The listing builds one solid part. Answer for the finished solid, in the listing's coordinates (mm). Coordinates: 2 decimals unless noted, no trailing zeros. Order: outer loops, then holes, each group sorted by start corner. A loop starts at its lowest first (then second) coordinate and runs counter-clockwise, first axis right, second up. Notation, with made-up numbers: (33, 55.5) -> (74, 55.5) arc R28 cw to (74, 81.5) -> close; hole circle Ø10 at (-3.5, 62.5). An arc over 180 degrees is marked (long way). Return JSON: item names as keys, results as strings.
```python
from build123d import *

# Parameters (mm, degrees)
F0_R     = 7.5
F1_DEPTH = 20


with BuildPart() as f1:
    # F0 (on Top) → F1 (new body)
    with BuildSketch(Plane.XY):
        with BuildLine():
            Line((-13.784993, 1.235994), (-16.59268, 2.329543))
            ThreePointArc((-16.59268, 2.329543), (-20, 0), (-16.59268, -2.329543))
            Line((-16.59268, -2.329543), (-13.784993, -1.235994))
            ThreePointArc((-13.784993, -1.235994), (-11.769423, -2.341084), (-13.208667, -4.133379))
            Line((-13.208667, -4.133379), (-16.221115, -4.197527))
            ThreePointArc((-16.221115, -4.197527), (-18.477591, -7.653669), (-14.43816, -8.501961))
            Line((-14.43816, -8.501961), (-12.262679, -6.417198))
            ThreePointArc((-12.262679, -6.417198), (-9.977635, -6.666843), (-10.621442, -8.873483))
            Line((-10.621442, -8.873483), (-13.380032, -10.085561))
            ThreePointArc((-13.380032, -10.085561), (-14.142136, -14.142136), (-10.085561, -13.380032))
            Line((-10.085561, -13.380032), (-8.873483, -10.621442))
            ThreePointArc((-8.873483, -10.621442), (-6.666843, -9.977635), (-6.417198, -12.262679))
            Line((-6.417198, -12.262679), (-8.501961, -14.43816))
            ThreePointArc((-8.501961, -14.43816), (-7.653669, -18.477591), (-4.197527, -16.221115))
            Line((-4.197527, -16.221115), (-4.133379, -13.208667))
            ThreePointArc((-4.133379, -13.208667), (-2.341084, -11.769423), (-1.235994, -13.784993))
            Line((-1.235994, -13.784993), (-2.329543, -16.59268))
            ThreePointArc((-2.329543, -16.59268), (0, -20), (2.329543, -16.59268))
            Line((2.329543, -16.59268), (1.235994, -13.784993))
            ThreePointArc((1.235994, -13.784993), (2.341084, -11.769423), (4.133379, -13.208667))
            Line((4.133379, -13.208667), (4.197527, -16.221115))
            ThreePointArc((4.197527, -16.221115), (7.653669, -18.477591), (8.501961, -14.43816))
            Line((8.501961, -14.43816), (6.417198, -12.262679))
            ThreePointArc((6.417198, -12.262679), (6.666843, -9.977635), (8.873483, -10.621442))
            Line((8.873483, -10.621442), (10.085561, -13.380032))
            ThreePointArc((10.085561, -13.380032), (14.142136, -14.142136), (13.380032, -10.085561))
            Line((13.380032, -10.085561), (10.621442, -8.873483))
            ThreePointArc((10.621442, -8.873483), (9.977635, -6.666843), (12.262679, -6.417198))
            Line((12.262679, -6.417198), (14.43816, -8.501961))
            ThreePointArc((14.43816, -8.501961), (18.477591, -7.653669), (16.221115, -4.197527))
            Line((16.221115, -4.197527), (13.208667, -4.133379))
            ThreePointArc((13.208667, -4.133379), (11.769423, -2.341084), (13.784993, -1.235994))
            Line((13.784993, -1.235994), (16.59268, -2.329543))
            ThreePointArc((16.59268, -2.329543), (20, 0), (16.59268, 2.329543))
            Line((16.59268, 2.329543), (13.784993, 1.235994))
            ThreePointArc((13.784993, 1.235994), (11.769423, 2.341084), (13.208667, 4.133379))
            Line((13.208667, 4.133379), (16.221115, 4.197527))
            ThreePointArc((16.221115, 4.197527), (18.477591, 7.653669), (14.43816, 8.501961))
            Line((14.43816, 8.501961), (12.262679, 6.417198))
            ThreePointArc((12.262679, 6.417198), (9.977635, 6.666843), (10.621442, 8.873483))
            Line((10.621442, 8.873483), (13.380032, 10.085561))
            ThreePointArc((13.380032, 10.085561), (14.142136, 14.142136), (10.085561, 13.380032))
            Line((10.085561, 13.380032), (8.873483, 10.621442))
            ThreePointArc((8.873483, 10.621442), (6.666843, 9.977635), (6.417198, 12.262679))
            Line((6.417198, 12.262679), (8.501961, 14.43816))
            ThreePointArc((8.501961, 14.43816), (7.653669, 18.477591), (4.197527, 16.221115))
            Line((4.197527, 16.221115), (4.133379, 13.208667))
            ThreePointArc((4.133379, 13.208667), (2.341084, 11.769423), (1.235994, 13.784993))
            Line((1.235994, 13.784993), (2.329543, 16.59268))
            ThreePointArc((2.329543, 16.59268), (0, 20), (-2.329543, 16.59268))
            Line((-2.329543, 16.59268), (-1.235994, 13.784993))
            ThreePointArc((-1.235994, 13.784993), (-2.341084, 11.769423), (-4.133379, 13.208667))
            Line((-4.133379, 13.208667), (-4.197527, 16.221115))
            ThreePointArc((-4.197527, 16.221115), (-7.653669, 18.477591), (-8.501961, 14.43816))
            Line((-8.501961, 14.43816), (-6.417198, 12.262679))
            ThreePointArc((-6.417198, 12.262679), (-6.666843, 9.977635), (-8.873483, 10.621442))
            Line((-8.873483, 10.621442), (-10.085561, 13.380032))
            ThreePointArc((-10.085561, 13.380032), (-14.142136, 14.142136), (-13.380032, 10.085561))
            Line((-13.380032, 10.085561), (-10.621442, 8.873483))
            ThreePointArc((-10.621442, 8.873483), (-9.977635, 6.666843), (-12.262679, 6.417198))
            Line((-12.262679, 6.417198), (-14.43816, 8.501961))
            ThreePointArc((-14.43816, 8.501961), (-18.477591, 7.653669), (-16.221115, 4.197527))
            Line((-16.221115, 4.197527), (-13.208667, 4.133379))
            ThreePointArc((-13.208667, 4.133379), (-11.769423, 2.341084), (-13.784993, 1.235994))
        make_face()
        Circle(F0_R, mode=Mode.SUBTRACT)
    extrude(amount=F1_DEPTH)


solid = f1.part
```
Item 1: The part is cut by section D-D on x = 8. Determine the outline of the cut face in (y, z), plus the area to 3 significant figures.
Answer list:
{"outline": "(-18.3, 0) -> (-13.91, 0) -> (-13.91, 20) -> (-18.3, 20) -> close; (-9.81, 0) -> (9.81, 0) -> (9.81, 20) -> (-9.81, 20) -> close; (13.91, 0) -> (18.3, 0) -> (18.3, 20) -> (13.91, 20) -> close", "area": "568 mm2"}
Item 2: Flat-ended cylindrical pins translate along their axes: pin 1 (10 mm diameter, centred on x = -3.5, y = 15.5, fed in from -Z); pin 2 (2 mm diameter, centred on x = -6.5, z = 15.5, fed in from -Y); pin 3 (10 mm diameter, centred on x = -6.5, z = 2.5, fed in from +Y); pin 4 (5 mm diameter, centred on y = 6, z = 15, fed in from -X). Find the tip coordinate at first contact, or state that the pin passes through.
Answer list:
{"pin 1": "z = 0", "pin 2": "y = -18.67", "pin 3": "y = 19.5", "pin 4": "x = -18.67"}
Item 3: The part is cut by section A-A on y = 0. Determine the outline of the cut face in (x, z), plus the area to 3 significant figures.
Answer list:
{"outline": "(-20, 0) -> (-7.5, 0) -> (-7.5, 20) -> (-20, 20) -> close; (7.5, 0) -> (20, 0) -> (20, 20) -> (7.5, 20) -> close", "area": "500 mm2"}
Item 4: The part is cut by section C-C on y = -17.5. Determine the outline of the cut face in (x, z).
Answer list:
{"outline": "(-8.81, 0) -> (-4.58, 0) -> (-4.58, 20) -> (-8.81, 20) -> close; (-2.5, 0) -> (2.5, 0) -> (2.5, 20) -> (-2.5, 20) -> close; (4.58, 0) -> (8.81, 0) -> (8.81, 20) -> (4.58, 20) -> close"}
Item 5: Find the intervals of material crossed by probe 1 along X at (y, z) = (-8.5, 8.25); probe 2 along X at (y, z) = (-9, 11); probe 3 along Y at (x, z) = (17.5, 15.25), in increasing order.
Answer list:
{"probe 1": "-17.9 to -14.44, -10.11 to 10.11, 14.44 to 17.9", "probe 2": "-17.14 to -15.2, -10.91 to 10.91, 15.2 to 17.14", "probe 3": "-8.81 to -4.58, -2.5 to 2.5, 4.58 to 8.81"}
